Design review of the part shown in the three views and the two pictorial views. Dimensions are in mm from the part's minimum x, y and z. A direction names the side the tool comes from. Give positions to 0.01 mm unless a question says otherwise; leave off trailing zeros. Write each loop counter-clockwise with the first axis right and the second up, starting at its lowest first coordinate (ties: lowest second). Pieces come first, ordered by that corner, then holes. Notation, with made-up numbers: M -27,-4.5 L 29,-4.5 A30 cw 29,21.5 Z; hole C 36,66.25 d6. An arc over 180 degrees is marked long. Write item = value, one per line.
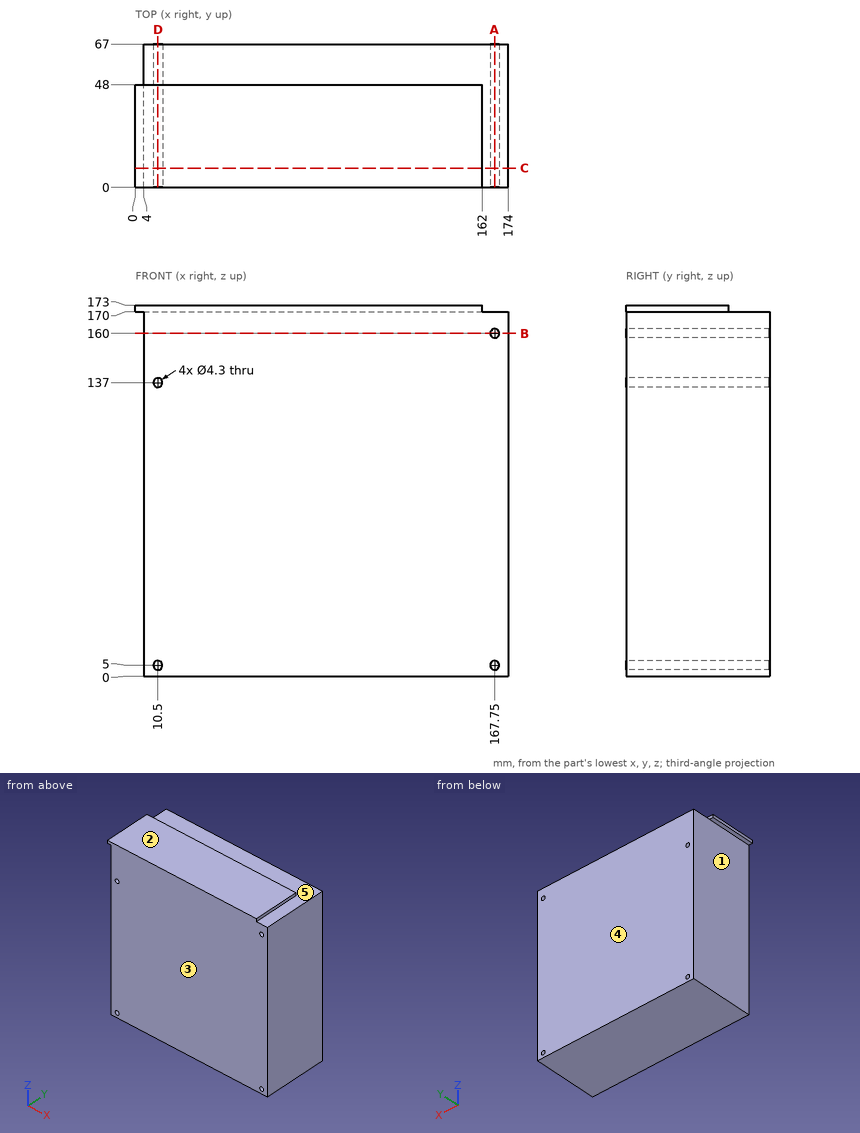
1. We need section A-A, the plane x = 167.75. Write out the cut boundary in (y, z), then the cut area to 3 significant figures.
Responses:
outline = M 0,0 L 67,0 L 67,2.85 L 0,2.85 Z; M 0,7.15 L 67,7.15 L 67,157.85 L 0,157.85 Z; M 0,162.15 L 67,162.15 L 67,170 L 0,170 Z
area = 10,800 mm2
2. For line 1 along Z through (x, y) = (10.5, 16); line 2 along X through (y, z) = (37, 5); line 3 along Z through (x, y) = (167.75, 25), list the stretches that pass through material, from the lowest coordinate up. Write a range as from..to.
Responses:
line_1 = 0..2.85, 7.15..134.85, 139.15..173
line_2 = 4..8.35, 12.65..165.6, 169.9..174
line_3 = 0..2.85, 7.15..157.85, 162.15..170
3. The part is to be moulded in two halves that separate along Y. For the marked faces 3, 4 and 5, say which applies: +Y half, -Y half, draft (parallel to the pull), parting line (faces both ways), or undercut.
Responses:
face_3 = -Y half
face_4 = +Y half
face_5 = draft
4. We need section D-D, the plane x = 10.5. Write out the cut boundary in (y, z), then the cut area to 3 significant figures.
Responses:
outline = M 0,0 L 67,0 L 67,2.85 L 0,2.85 Z; M 0,7.15 L 67,7.15 L 67,134.85 L 0,134.85 Z; M 0,139.15 L 67,139.15 L 67,170 L 48,170 L 48,173 L 0,173 Z
area = 11,000 mm2
5. Insertion check: P1, Ø2, axis at x = 148, y = 58, coming from the +Z side; P2, Ø0.9, axis at x = 78.5, z = 171, coming from the +Y side; P3, Ø8, axis at y = 44.5, z = 114.5, coming from the -X side. Each pin has a flat end and moves straight along its axis. Give the tip position at first contact, or say it passes through.
Responses:
P1 = 170
P2 = 48
P3 = 4
6. We need section B-B, the plane z = 160. Write out the cut boundary in (x, y).
Responses:
outline = M 4,0 L 165.6,0 L 165.6,67 L 4,67 Z; M 169.9,0 L 174,0 L 174,67 L 169.9,67 Z
7. Machinability: for the marked faces 1 and 2, which of the approach directions +Z, -Z, +X, -X, +Y, -Y give a long, thin tool a straight path to every point of the face, cutting with its end or side? Answer none if there is none.
Responses:
face_1 = -Z, -X, +Y, -Y
face_2 = +Z, +X, -X, +Y, -Y
8. We need section C-C, the plane y = 9. Write out the cut boundary in (x, z), then the cut area to 3 significant figures.
Responses:
outline = M 0,170 L 4,170 L 4,0 L 174,0 L 174,170 L 162,170 L 162,173 L 0,173 Z; hole C 10.5,5 d4.3; hole C 10.5,137 d4.3; hole C 167.75,5 d4.3; hole C 167.75,160 d4.3
area = 29,300 mm2
